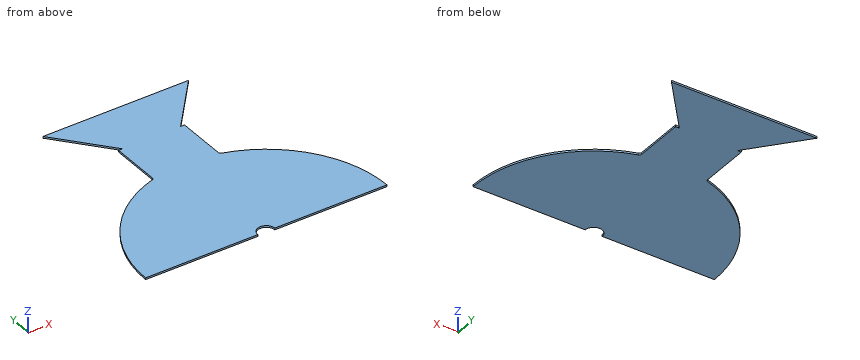
from build123d import *

# Parameters (mm, degrees)
BASE_FLANGE1_DEPTH = 2.65684
FILLET1_R          = 3.175


# Sheet-metal steps are written as plain solids
with BuildPart() as part:
    # Sketch1 → Base-Flange1 (new body)
    with BuildSketch(Plane.XY):
        with BuildLine():
            Line((-180.45684, 0), (-12.7, 0))
            ThreePointArc((-12.7, 0), (0, 12.7), (12.7, 0))
            Line((12.7, 0), (180.45684, 0))
            ThreePointArc((180.45684, 0), (143.97849234, 108.788165011), (49.29124, 173.594483674))
            Line((49.29124, 173.594483674), (49.29124, 249.794483674))
            Line((49.29124, 249.794483674), (43.488704599, 249.794483674))
            Line((43.488704599, 249.794483674), (108.795925743, 327.624599095))
            Line((108.795925743, 327.624599095), (-108.795925743, 327.624599095))
            Line((-108.795925743, 327.624599095), (-43.488704599, 249.794483674))
            Line((-43.488704599, 249.794483674), (-49.29124, 249.794483674))
            Line((-49.29124, 249.794483674), (-49.29124, 173.594483674))
            ThreePointArc((-49.29124, 173.594483674), (-143.97849234, 108.788165011), (-180.45684, 0))
        make_face()
    extrude(amount=-BASE_FLANGE1_DEPTH)

    # Fillet1
    fillet1_edges = [part.edges().sort_by_distance(p)[0] for p in [
        (-49.29124, 173.594483674, -1.32842),
        (49.29124, 173.594483674, -1.32842),
    ]]
    fillet(fillet1_edges, radius=FILLET1_R)


solid = part.part
The listing builds one solid part. Answer for the finished solid, in the listing's coordinates (mm). Coordinates: 2 decimals unless noted, no trailing zeros. Loops run counter-clockwise (first coordinate to the right, second up) from the corner with the lowest first, then second, coordinate; pieces in that order, holes last. Notation, with made-up numbers: (76, -38.5) -> (125, -38.5) arc R28 ccw to (125, -12.5) -> close; hole circle Ø7 at (81, 58.5). An arc over 180 degrees is marked (long way). Write item = value, one per line. Start each with the question number.
1) Given pin 1 Ø1 at (x, y) = (-13.5, 141.5) entering from +Z; pin 2 Ø1 at (y, z) = (260.5, -0.5) entering from -X, each flat-ended and moving along its own axis, determine where each tip first touches the part or whether it passes through.
2) A cutting plane is placed at C-C (y = 274). Give the vertices of the cut face in (x, z).
3) A cutting plane is placed at B-B (x = 0). Give the vertices of the cut face in (y, z), then the cut area to 3 significant figures.
4) Straight lines are drawn through the part: line 1 (X direction, y = 205, z = -2.5); line 2 (Y direction, x = 50, z = -1.15); line 3 (Y direction, x = -105.5, z = -2.05) (3 decimals). For each, find the intervals that lie inside material, in ascending order. Write a range as from..to.
5) A cutting plane is placed at A-A (z = -1.05). Give the vertices of the cut face in (x, y) (3 decimals), then the cut area to 3 significant figures.
Responses:
q1.pin_1 = 0
q1.pin_2 = -52.89
q2.outline = (-63.8, -2.66) -> (63.8, -2.66) -> (63.8, 0) -> (-63.8, 0) -> close
q3.outline = (12.7, -2.66) -> (327.62, -2.66) -> (327.62, 0) -> (12.7, 0) -> close
q3.area = 837 mm²
q4.line_1 = -49.29..49.29
q4.line_2 = 0..173.98, 257.55..327.62
q4.line_3 = 0..146.405, 323.697..327.625
q5.outline = (-180.457, 0) -> (-12.7, 0) arc R12.7 cw to (12.7, 0) -> (180.457, 0) arc R180.457 ccw to (51.559, 172.934) arc R3.175 cw to (49.291, 175.977) -> (49.291, 249.794) -> (43.489, 249.794) -> (108.796, 327.625) -> (-108.796, 327.625) -> (-43.489, 249.794) -> (-49.291, 249.794) -> (-49.291, 175.977) arc R3.175 cw to (-51.559, 172.934) arc R180.457 ccw to start
q5.area = 69,800 mm²
